Here's how the part is built. I have some questions about the finished solid (model axes, mm). Face numbers are marked on the shaded views. A direction names the side the tool comes from. Round coordinates to 2 decimals unless told otherwise and drop trailing zeros. Loops run counter-clockwise (first coordinate to the right, second up) from the corner with the lowest first, then second, coordinate; pieces in that order, holes last. Notation, with made-up numbers: M 57,-34 L 66,-34 A14 ccw 66,-21 Z; hole C 12,-32 d4. An arc over 180 degrees is marked long. Use a Markdown table: item, result.
```python
from build123d import *

# Parameters (mm, degrees)
SKETCH_1_W          = 160
SKETCH_1_H          = 150
EXTRUDE_1_DEPTH     = 3
SKETCH_2_W          = 160
SKETCH_2_H          = 92.8
SKETCH_2_W_2        = 150
SKETCH_2_H_2        = 87
EXTRUDE_2_DEPTH     = 80
SKETCH_4_W          = 45
SKETCH_4_H          = 29
CUT_EXTRUDE_2_DEPTH = 3


with BuildPart() as part:
    # ｽｹｯﾁ1 → ﾎﾞｽ - 押し出し1 (new body)
    with BuildSketch(Plane.XY):
        Rectangle(SKETCH_1_W, SKETCH_1_H)
    extrude(amount=EXTRUDE_1_DEPTH)

    # ｽｹｯﾁ2 → ﾎﾞｽ - 押し出し2 (add)
    with BuildSketch(Plane.XY.offset(3)):
        with Locations((0, -13.6)):
            Rectangle(SKETCH_2_W, SKETCH_2_H)
        with Locations((0, -13.6)):
            Rectangle(SKETCH_2_W_2, SKETCH_2_H_2, mode=Mode.SUBTRACT)
    extrude(amount=EXTRUDE_2_DEPTH)

    # ｽｹｯﾁ4 → ｶｯﾄ - 押し出し2 (cut)
    with BuildSketch(Plane.XY.offset(3)):
        with Locations((-57.5, 60.5)):
            Rectangle(SKETCH_4_W, SKETCH_4_H)
        with Locations((57.5, 60.5)):
            Rectangle(SKETCH_4_W, SKETCH_4_H)
    extrude(amount=-CUT_EXTRUDE_2_DEPTH, mode=Mode.SUBTRACT)


solid = part.part
```
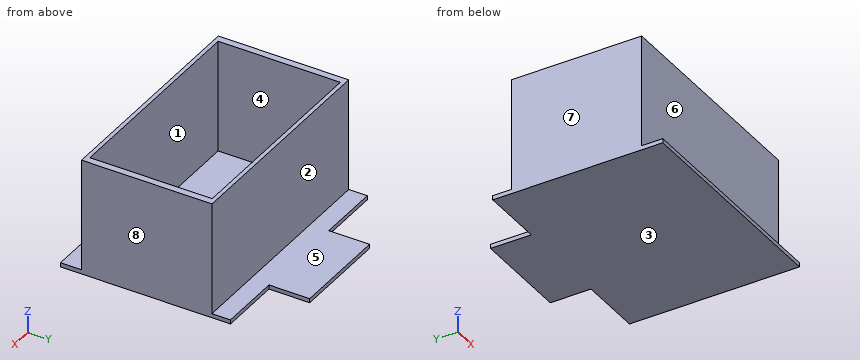
Q1. Imagine slicing it at C-C, the plane x = 1.5. Please give me the cut outline in (y, z).
Return value:
| item | result |
|---|---|
| outline | M -75,0 L 75,0 L 75,3 L 32.8,3 L 32.8,83 L 29.9,83 L 29.9,3 L -57.1,3 L -57.1,83 L -60,83 L -60,3 L -75,3 Z |
Q2. Will these pins go through, and if not, where does the flat tip stop? P1, Ø4.5, axis at x = -33.5, y = -64.5, coming from the +Z side; P2, Ø1.5, axis at x = 63.5, z = 2, coming from the +Y side; P3, Ø8, axis at x = 56, z = 10.5, coming from the +Y side.
Return value:
| item | result |
|---|---|
| P1 | stops at z = 3 |
| P2 | stops at y = 46 |
| P3 | stops at y = 32.8 |
Q3. We'd pull the mould along Y, two halves only. Please class the marked faces 1, 2 and 3: pulls with the +Y half, pulls with the -Y half, needs draft (parallel to the pull), parting line crosses it, or undercut.
Return value:
| item | result |
|---|---|
| face 1 | undercut |
| face 2 | pulls with the +Y half |
| face 3 | needs draft |
Q4. Imagine slicing it at B-B, the plane z = 41. Please give me the cut outline in (x, y).
Return value:
| item | result |
|---|---|
| outline | M -80,-60 L 80,-60 L 80,32.8 L -80,32.8 Z; hole M -75,-57.1 L 75,-57.1 L 75,29.9 L -75,29.9 Z |
Q5. Imagine slicing it at D-D, the plane x = -65.5. Please give me the cut outline in (y, z).
Return value:
| item | result |
|---|---|
| outline | M -75,0 L 46,0 L 46,3 L 32.8,3 L 32.8,83 L 29.9,83 L 29.9,3 L -57.1,3 L -57.1,83 L -60,83 L -60,3 L -75,3 Z |
Q6. I need wall thicknesses on line 1 (Y direction, x = -17, z = 14); line 2 (X direction, y = -43, z = 37.5); line 3 (Z direction, x = 4.5, y = 11). Which ranges of each line are inside material? Lowest first, please. Write a range as from..to.
Return value:
| item | result |
|---|---|
| line 1 | y = -60..-57.1, 29.9..32.8 |
| line 2 | x = -80..-75, 75..80 |
| line 3 | z = 0..3 |
Q7. Imagine slicing it at A-A, the plane y = 16.5. Please give me the cut outline in (x, z).
Return value:
| item | result |
|---|---|
| outline | M -80,0 L 80,0 L 80,83 L 75,83 L 75,3 L -75,3 L -75,83 L -80,83 Z |
Q8. For the marked faces 4, 5, 6, 7 and 8, which set-ups out of +Z, -Z, +X, -X, +Y, -Y let a thin tool reach every point of the face, with its end or its side?
Return value:
| item | result |
|---|---|
| face 4 | +Z |
| face 5 | +Z, +X, -X, +Y |
| face 6 | +Z, +X, -X, -Y |
| face 7 | +Z, -Z, -X, +Y, -Y |
| face 8 | +Z, -Z, +X, +Y, -Y |
